Input: part model. Units: mm. Frame: model coordinates. A direction names the side the tool comes from. Round coordinates to 2 decimals unless told otherwise and drop trailing zeros. Order: outer loops, then holes, each group sorted by start corner. A loop starts at its lowest first (then second) coordinate and runs counter-clockwise, first axis right, second up. Notation, with made-up numbers: M -20.5,-21.5 L 28.5,-21.5 A27 ccw 28.5,10.5 Z; hole C 87.5,-14.75 d9. An arc over 180 degrees is marked long. One line per question, with ' | ' between items.
```python
from build123d import *

# Parameters (mm, degrees)
SKETCH1_W           = 125
SKETCH1_H           = 50.8
BOSS_EXTRUDE1_DEPTH = 3.175
SKETCH2_R           = 8.255
CUT_EXTRUDE1_DEPTH  = 135.965627569
SKETCH3_W           = 9.4
SKETCH3_H           = 50.8
CUT_EXTRUDE2_DEPTH  = 10


with BuildPart() as part:
    # Sketch1 → Boss-Extrude1 (new body)
    with BuildSketch(Plane(origin=(0, 0, 0), x_dir=(1, 0, 0), z_dir=(0, 1, 0))):
        with Locations((62.5, 25.4)):
            Rectangle(SKETCH1_W, SKETCH1_H)
    extrude(amount=BOSS_EXTRUDE1_DEPTH)

    # Sketch2 → Cut-Extrude1 (cut, through all)
    with BuildSketch(Plane(origin=(0, 3.175, 0), x_dir=(1, 0, 0), z_dir=(0, 1, 0))):
        with Locations(Location((99.6, 25.4, 0), (0, 0, 270))):
            Circle(SKETCH2_R)
        with BuildLine():
            Line((3.175, 42.2), (8.175, 42.2))
            ThreePointArc((8.175, 42.2), (10.425, 44.45), (8.175, 46.7))
            Line((8.175, 46.7), (3.175, 46.7))
            ThreePointArc((3.175, 46.7), (0.925, 44.45), (3.175, 42.2))
        make_face()
        with BuildLine():
            Line((3.175, 4.1), (8.175, 4.1))
            ThreePointArc((8.175, 4.1), (10.425, 6.35), (8.175, 8.6))
            Line((8.175, 8.6), (3.175, 8.6))
            ThreePointArc((3.175, 8.6), (0.925, 6.35), (3.175, 4.1))
        make_face()
        with BuildLine():
            Line((80.425, 40.35), (85.425, 40.35))
            ThreePointArc((85.425, 40.35), (87.675, 38.1), (85.425, 35.85))
            Line((85.425, 35.85), (80.425, 35.85))
            Line((80.425, 35.85), (75.425, 35.85))
            ThreePointArc((75.425, 35.85), (73.175, 38.1), (75.425, 40.35))
            Line((75.425, 40.35), (80.425, 40.35))
        make_face()
        with BuildLine():
            Line((48.8, 35.85), (43.8, 35.85))
            ThreePointArc((43.8, 35.85), (41.55, 38.1), (43.8, 40.35))
            Line((43.8, 40.35), (48.8, 40.35))
            Line((48.8, 40.35), (53.8, 40.35))
            ThreePointArc((53.8, 40.35), (56.05, 38.1), (53.8, 35.85))
            Line((53.8, 35.85), (48.8, 35.85))
        make_face()
        with BuildLine():
            Line((48.8, 10.45), (43.8, 10.45))
            ThreePointArc((43.8, 10.45), (41.55, 12.7), (43.8, 14.95))
            Line((43.8, 14.95), (48.8, 14.95))
            Line((48.8, 14.95), (53.8, 14.95))
            ThreePointArc((53.8, 14.95), (56.05, 12.7), (53.8, 10.45))
            Line((53.8, 10.45), (48.8, 10.45))
        make_face()
        with BuildLine():
            Line((80.425, 10.45), (75.425, 10.45))
            ThreePointArc((75.425, 10.45), (73.175, 12.7), (75.425, 14.95))
            Line((75.425, 14.95), (80.425, 14.95))
            Line((80.425, 14.95), (85.425, 14.95))
            ThreePointArc((85.425, 14.95), (87.675, 12.7), (85.425, 10.45))
            Line((85.425, 10.45), (80.425, 10.45))
        make_face()
    extrude(amount=-CUT_EXTRUDE1_DEPTH, mode=Mode.SUBTRACT)

    # Sketch3 → Cut-Extrude2 (cut)
    with BuildSketch(Plane(origin=(0, 3.175, 0), x_dir=(1, 0, 0), z_dir=(0, 1, 0))):
        with Locations((120.3, 25.4)):
            Rectangle(SKETCH3_W, SKETCH3_H)
    extrude(amount=-CUT_EXTRUDE2_DEPTH, mode=Mode.SUBTRACT)


solid = part.part
```
Item 1: Section query B-B, the plane x = 45.5. Return loops of the section in (y, z) (3 decimals), plus the area to 3 significant figures.
Report:
outline: M 0,-50.8 L 3.175,-50.8 L 3.175,-40.35 L 0,-40.35 Z; M 0,-35.85 L 3.175,-35.85 L 3.175,-14.95 L 0,-14.95 Z; M 0,-10.45 L 3.175,-10.45 L 3.175,0 L 0,0 Z | area: 133 mm²
Item 2: Section query D-D, the plane z = -25.4. Return loops of the section in (x, y) (3 decimals).
Report:
outline: M 0,0 L 91.345,0 L 91.345,3.175 L 0,3.175 Z; M 107.855,0 L 115.6,0 L 115.6,3.175 L 107.855,3.175 Z
Item 3: Access query for faces 5 (the flat face through (80, 2, -10.45)), 6 (the flat face through (57, 2, -50.8)). Directions: +Z, -Z, +X, -X, +Y, -Y. A direction counts if a zero-diameter tool reaches every point of the face in a straight line with its end or side. Return the directions, or none.
Report:
face 5: +Y, -Y | face 6: -Z, +X, -X, +Y, -Y
Item 4: Line query: line 1 along Z through (x, y) = (50, 0.85); line 2 along X through (y, z) = (0.85, -25.4) (3 decimals); line 3 along X through (y, z) = (0.3, -12). Output: solid intervals per line, ascending. Write a range as from..to.
Report:
line 1: -50.8..-40.35, -35.85..-14.95, -10.45..0 | line 2: 0..91.345, 107.855..115.6 | line 3: 0..41.66, 55.94..73.29, 87.56..115.6
Item 5: Mould query, pull axis X, two halves, no side actions, for faces 1 (the flat face through (57, 0, -26)), 2 (the cylindrical face through (41.55, 1.61, -38.05)), 3 (the flat face through (0, 2, -25)), 4 (the cylindrical face through (87.674, 1.61, -12.749)). Classes: +X half, -X half, draft (parallel to the pull), parting line (faces both ways), or undercut.
Report:
face 1: draft | face 2: undercut | face 3: -X half | face 4: undercut
Item 6: Section query C-C, the plane z = -38.1. Return loops of the section in (x, y) (3 decimals).
Report:
outline: M 0,0 L 41.55,0 L 41.55,3.175 L 0,3.175 Z; M 56.05,0 L 73.175,0 L 73.175,3.175 L 56.05,3.175 Z; M 87.675,0 L 115.6,0 L 115.6,3.175 L 87.675,3.175 Z
Item 7: Section query A-A, the plane z = -44.45. Return loops of the section in (x, y) (3 decimals).
Report:
outline: M 0,0 L 0.925,0 L 0.925,3.175 L 0,3.175 Z; M 10.425,0 L 115.6,0 L 115.6,3.175 L 10.425,3.175 Z
